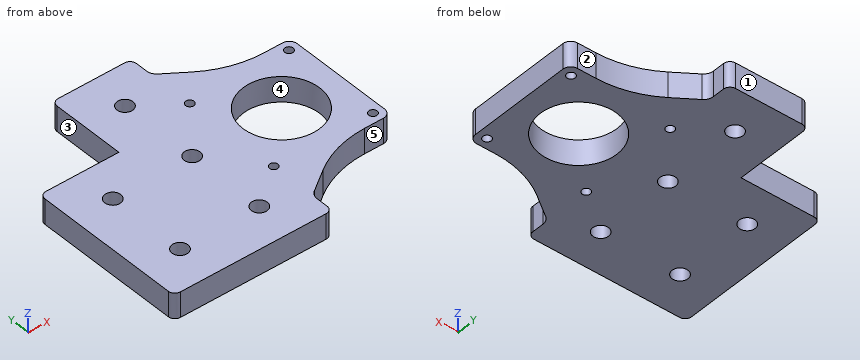
from build123d import *

# Parameters (mm, degrees)
SKETCH1_R                = 4
SKETCH1_R_2              = 13.05
BOSS_EXTRUDE1_DEPTH      = 12.7
BOSS_EXTRUDE2_START      = -3.2
SKETCH2_R                = 13.05
SKETCH2_R_2              = 10
BOSS_EXTRUDE2_DEPTH      = 3.2
FILLET1_R                = 5
FILLET2_R                = 3.25
BOSS_EXTRUDE3_START      = -12.7
BOSS_EXTRUDE3_DEPTH      = 12.7
CUT_EXTRUDE1_START       = -12.7
CUT_EXTRUDE1_OUTLINE_R   = 19.275
CUT_EXTRUDE1_OUTLINE_R_2 = 10
CUT_EXTRUDE1_DEPTH       = 12.7
FILLET3_R                = 4
FILLET4_R                = 50
M5X0_8_TAPPED_HOLE1_D    = 4.2


# Read off the part's stored shape, not the designer's step: Boss-Extrude3, Cut-Extrude1
with BuildPart() as part:
    # Sketch1 → Boss-Extrude1 (new body)
    with BuildSketch(Plane.XY):
        with BuildLine():
            Line((0, 0), (0, 11.914408096))
            Line((0, 11.914408096), (39.368089731, 39.480241291))
            ThreePointArc((39.368089731, 39.480241291), (50.05, 60), (39.368089731, 80.519758709))
            Line((39.368089731, 80.519758709), (0, 108.085591904))
            Line((0, 108.085591904), (0, 120))
            Line((0, 120), (-40, 120))
            Line((-40, 120), (-40, 80))
            Line((-40, 80), (-80, 80))
            Line((-80, 80), (-80, 0))
            Line((-80, 0), (0, 0))
        make_face()
        with Locations((-20, 20)):
            Circle(SKETCH1_R, mode=Mode.SUBTRACT)
        with Locations((-60, 20)):
            Circle(SKETCH1_R, mode=Mode.SUBTRACT)
        with Locations((-60, 60)):
            Circle(SKETCH1_R, mode=Mode.SUBTRACT)
        with Locations((-20, 60)):
            Circle(SKETCH1_R, mode=Mode.SUBTRACT)
        with Locations((-20, 100)):
            Circle(SKETCH1_R, mode=Mode.SUBTRACT)
        with Locations((25, 60)):
            Circle(SKETCH1_R_2, mode=Mode.SUBTRACT)
    extrude(amount=BOSS_EXTRUDE1_DEPTH)

    # Sketch2 → Boss-Extrude2 (add)
    with BuildSketch(Plane.XY.offset(12.7).offset(BOSS_EXTRUDE2_START)):
        with Locations((25, 60)):
            Circle(SKETCH2_R)
        with Locations((25, 60)):
            Circle(SKETCH2_R_2, mode=Mode.SUBTRACT)
    extrude(amount=BOSS_EXTRUDE2_DEPTH)

    # Fillet1
    fillet1_edges = [part.edges().sort_by_distance(p)[0] for p in [
        (0, 108.085591904, 6.35),
        (0, 11.914408096, 6.35),
    ]]
    fillet(fillet1_edges, radius=FILLET1_R)

    # Fillet2
    fillet2_edges = [part.edges().sort_by_distance(p)[0] for p in [
        (-80, 0, 6.35),
        (-80, 80, 6.35),
        (-40, 120, 6.35),
        (0, 120, 6.35),
        (0, 0, 6.35),
    ]]
    fillet(fillet2_edges, radius=FILLET2_R)

    # Boss-Extrude3 outline → Boss-Extrude3 (add)
    with BuildSketch(Plane(origin=(0, 0, 0), x_dir=(-1, 0, 0), z_dir=(0, 0, -1)).offset(BOSS_EXTRUDE3_START)):
        with BuildLine():
            Line((-55, 90), (-55, 30))
            Line((-55, 30), (-25.828902028, 30))
            Line((-25.828902028, 30), (-39.368089731, 39.480241291))
            ThreePointArc((-39.368089731, 39.480241291), (-50.05, 60), (-39.368089731, 80.519758709))
            Line((-39.368089731, 80.519758709), (-25.828902028, 90))
            Line((-25.828902028, 90), (-55, 90))
        make_face()
    extrude(amount=BOSS_EXTRUDE3_DEPTH)

    # Cut-Extrude1 outline → Cut-Extrude1 (cut)
    with BuildSketch(Plane(origin=(0, 0, 0), x_dir=(-1, 0, 0), z_dir=(0, 0, -1)).offset(CUT_EXTRUDE1_START)):
        with Locations((-25, 60)):
            Circle(CUT_EXTRUDE1_OUTLINE_R)
        with Locations((-25, 60)):
            Circle(CUT_EXTRUDE1_OUTLINE_R_2, mode=Mode.SUBTRACT)
    extrude(amount=CUT_EXTRUDE1_DEPTH, mode=Mode.SUBTRACT)

    # Fillet3
    fillet3_edges = [part.edges().sort_by_distance(p)[0] for p in [
        (55, 90, 6.35),
        (55, 30, 6.35),
    ]]
    fillet(fillet3_edges, radius=FILLET3_R)

    # Fillet4
    fillet4_edges = [part.edges().sort_by_distance(p)[0] for p in [
        (25.828902028, 30, 6.35),
        (25.828902028, 90, 6.35),
    ]]
    fillet(fillet4_edges, radius=FILLET4_R)

    # M5x0.8 Tapped Hole1 (through all)
    with Locations(Plane(origin=(0, 0, 0), x_dir=(-1, 0, 0), z_dir=(0, 0, -1))):
        with Locations((0, 85), (0, 35), (-50, 85), (-50, 35)):
            Hole(M5X0_8_TAPPED_HOLE1_D / 2)


solid = part.part
Work out the finished part from the listing and answer in its coordinate system (mm). Face numbers are marked on the shaded views. A direction names the side the tool comes from. Coordinates: 2 decimals unless noted, no trailing zeros. Write each loop counter-clockwise with the first axis right and the second up, starting at its lowest first coordinate (ties: lowest second). Pieces come first, ordered by that corner, then holes. Notation, with made-up numbers: M -26.75,39.5 L 15.25,39.5 A20 ccw 15.25,51.5 Z; hole C 11,10.5 d7. An arc over 180 degrees is marked long. Use one line per item in the form item = value. Start each with the question number.
1. A tool of negligible diameter and unlimited length cuts with its end or side. For the marked faces 1, 2, 3, 4 and 5, from which of +Z, -Z, +X, -X, +Y, -Y can it reach the whole face along a straight path? Write none if from no direction.
2. The part is cut by section B-B (x = -19.5). Give the vertices of the cut face in (y, z), plus the area to 3 significant figures.
3. Each of these flat-tipped pins is pushed along its axis until it touches: P1, Ø3, axis at x = 48, z = 5.5, coming from the +Y side; P2, Ø1.5, axis at y = 90, z = 3, coming from the -X side; P3, Ø4.5, axis at x = 44.5, z = 3.5, coming from the -Y side; P4, Ø2.5, axis at x = 0, y = 85, coming from the -Z side. Where does it stop, or does it pass through?
4. Straight lines are drawn through the part: probe 1 along Y at (x, z) = (-20, 7.5); probe 2 along Y at (x, z) = (50, 7.25); probe 3 along Y at (x, z) = (-60, 9.5). For each, find the intervals that lie inside material, in ascending order. Write a range as from..to.
5. The part is cut by section A-A (y = 60). Give the vertices of the cut face in (x, z) (3 decimals).
6. The part is cut by section D-D (x = 25). Give the vertices of the cut face in (y, z) (3 decimals), plus the area to 3 significant figures.
7. The part is cut by section C-C (z = 1.5). Give the number of separate pieces and of enclosed holes in the cut face, plus the area to 3 significant figures.
Evaluation:
q1.face_1 = +Z, -Z, +X, -X, +Y
q1.face_2 = +Z, -Z, +X, +Y
q1.face_3 = +Z, -Z, -X, +Y
q1.face_4 = +Z, -Z
q1.face_5 = +Z, -Z, +X, -Y
q2.outline = M 0,0 L 16.03,0 L 16.03,12.7 L 0,12.7 Z; M 23.97,0 L 56.03,0 L 56.03,12.7 L 23.97,12.7 Z; M 63.97,0 L 96.03,0 L 96.03,12.7 L 63.97,12.7 Z; M 103.97,0 L 120,0 L 120,12.7 L 103.97,12.7 Z
q2.area = 1,220 mm^2
q3.P1 = 90
q3.P2 = -40
q3.P3 = 30
q3.P4 = through
q4.probe_1 = 0..16, 24..56, 64..96, 104..120
q4.probe_2 = 30..32.9, 37.1..82.9, 87.1..90
q4.probe_3 = 0..16, 24..56, 64..80
q5.outline = M -80,0 L -64,0 L -64,12.7 L -80,12.7 Z; M -56,0 L -24,0 L -24,12.7 L -56,12.7 Z; M -16,0 L 5.725,0 L 5.725,12.7 L -16,12.7 Z; M 44.275,0 L 55,0 L 55,12.7 L 44.275,12.7 Z
q6.outline = M 27.166,0 L 40.725,0 L 40.725,12.7 L 27.166,12.7 Z; M 79.275,0 L 92.834,0 L 92.834,12.7 L 79.275,12.7 Z
q6.area = 344 mm^2
q7.separate_pieces = 1
q7.enclosed_holes = 10
q7.area = 10,300 mm^2
